Build history of the part. All positions in model axes, mm. Face numbers are marked on the shaded views. A direction names the side the tool comes from. Give positions to 0.01 mm unless a question says otherwise; leave off trailing zeros. Loops run counter-clockwise (first coordinate to the right, second up) from the corner with the lowest first, then second, coordinate; pieces in that order, holes last.
1) Band-saw the part on A-A on y = 1.5. List the corners of the cut face in (x, z).
2) 3-axis set-ups, long thin cutter, end or side, ignore diameter. For the marked faces 1 and 2: which of +Z, -Z, +X, -X, +Y, -Y reach the whole face in a straight line?
3) Flat gauge pins, fed straight in: P1, Ø1, axis at x = 73, y = -1, coming from the -Z side; P2, Ø1.5, axis at x = 96.5, y = 0.5, coming from the -Z side. Where does each tip first touch, or does it go through?
4) Wall check: line 1 (X direction, y = 3.25, z = 1); line 2 (Z direction, x = 87.5, y = 0); line 3 (Z direction, x = 76, y = 1). Give the ranges that are in metal, low to high.
5) Band-saw the part on C-C on x = 19.5. List the corners of the cut face in (y, z), then the cut area to 3 significant figures.
Autodesk Inventor part; units mm, degrees
ref_plane "YZ Plane" through (0, 0, 0) normal (1, 0, 0) x (0, 1, 0)
ref_plane "XZ Plane" through (0, 0, 0) normal (0, 1, 0) x (-1, 0, 0)
ref_plane "XY Plane" through (0, 0, 0) normal (0, 0, 1) x (1, 0, 0)
sketch "Sketch1" plane through (0, 0, 0) normal (1, 0, 0) x (0, 1, 0)
  circle A0 centre (0, 0) radius 2.5
  dimension "d0" = 5
extrude "Extrusion1" add sketch "Sketch1" along normal blind 110
sketch "Sketch2" plane through (110, 0, 0) normal (1, 0, 0) x (0, 0, -1)
  circle A0 centre (0, 0) radius 2.5 construction
  line L0 (4, 4) -> (-4, 4)
  line L1 (-4, 4) -> (-4, -4)
  line L2 (-4, -4) -> (4, -4)
  line L3 (4, -4) -> (4, 4)
  line L4 (4, 4) -> (-4, -4) construction
  line L5 (-4, 4) -> (4, -4) construction
  dimension "d5" = 8
  dimension "d6" = 8
extrude "Extrusion2" add sketch "Sketch2" along normal blind 2
properties part number "shaft"
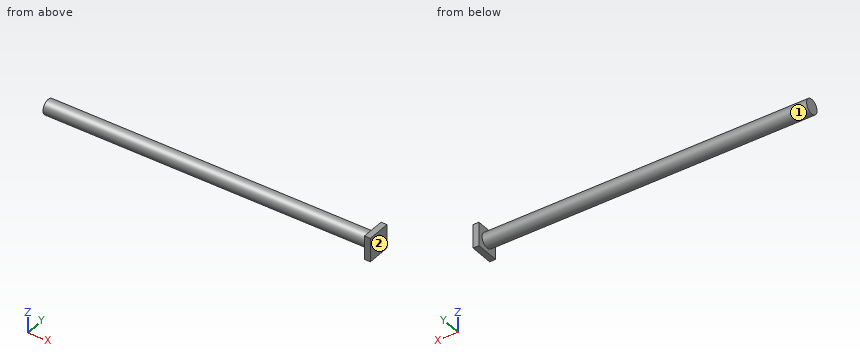
Findings below:
1. outline: (0, -2) - (110, -2) - (110, -4) - (112, -4) - (112, 4) - (110, 4) - (110, 2) - (0, 2) - close
2. face 1: -X
2. face 2: +Z, -Z, +X, +Y, -Y
3. P1: stops at z = -2.45
3. P2: stops at z = -2.5
4. line 1: x = 110 to 112
4. line 2: z = -2.5 to 2.5
4. line 3: z = -2.29 to 2.29
5. outline: circle Ø5 at (0, 0)
5. area: 19.6 mm2
